```python
from build123d import *

# Parameters (mm, degrees)
SKETCH1_W           = 85
SKETCH1_H           = 70
SKETCH1_R           = 1.375
SKETCH1_R_2         = 4.125
SKETCH1_W_2         = 2.024682369
SKETCH1_H_2         = 6.385975888
SKETCH1_R_3         = 1.875
SKETCH1_R_4         = 2
SKETCH1_R_5         = 3
BOSS_EXTRUDE4_DEPTH = 10
SKETCH1_7_R         = 4.5
CUT_EXTRUDE2_DEPTH  = 6
SKETCH1_11_R        = 4.5
SKETCH1_11_R_2      = 3
CUT_EXTRUDE10_DEPTH = 8


with BuildPart() as part:
    # Sketch1 → Boss-Extrude4 (new body)
    with BuildSketch(Plane(origin=(0, 0, 0), x_dir=(1, 0, 0), z_dir=(0, 1, 0))):
        with Locations((-9.775924906, 0)):
            Rectangle(SKETCH1_W, SKETCH1_H)
        with Locations((-37.275924906, -25)):
            Circle(SKETCH1_R, mode=Mode.SUBTRACT)
        with Locations((12.724075094, -25)):
            Circle(SKETCH1_R, mode=Mode.SUBTRACT)
        with Locations((-25.024682369, 0)):
            Circle(SKETCH1_R_2, mode=Mode.SUBTRACT)
        with Locations((-18.012341185, 0)):
            Rectangle(SKETCH1_W_2, SKETCH1_H_2, mode=Mode.SUBTRACT)
        with Locations((-37.275924906, 25)):
            Circle(SKETCH1_R, mode=Mode.SUBTRACT)
        with Locations((12.724075094, 25)):
            Circle(SKETCH1_R, mode=Mode.SUBTRACT)
        with Locations((0, 17.5)):
            Circle(SKETCH1_R_3, mode=Mode.SUBTRACT)
        with Locations((0, -17.5)):
            Circle(SKETCH1_R_4, mode=Mode.SUBTRACT)
        with Locations((7, 0)):
            Circle(SKETCH1_R_5, mode=Mode.SUBTRACT)
    extrude(amount=BOSS_EXTRUDE4_DEPTH)

    # Sketch1_7 → Cut-Extrude2 (cut)
    with BuildSketch(Plane(origin=(0, 0, 0), x_dir=(1, 0, 0), z_dir=(0, 1, 0))):
        with BuildLine():
            Line((3.625, 17.5), (3.625, 13.729507457))
            ThreePointArc((3.625, 13.729507457), (14.2, 0), (3.625, -13.729507457))
            Line((3.625, -13.729507457), (3.625, -17.5))
            ThreePointArc((3.625, -17.5), (0, -21.125), (-3.625, -17.5))
            Line((-3.625, -17.5), (-3.625, -13.729507457))
            ThreePointArc((-3.625, -13.729507457), (-8.669470541, -11.246345208), (-12.354756169, -7))
            Line((-12.354756169, -7), (-17, -7))
            Line((-17, -7), (-17, 7))
            Line((-17, 7), (-12.354756169, 7))
            ThreePointArc((-12.354756169, 7), (-8.669470541, 11.246345208), (-3.625, 13.729507457))
            Line((-3.625, 13.729507457), (-3.625, 17.5))
            ThreePointArc((-3.625, 17.5), (0, 21.125), (3.625, 17.5))
        make_face()
        with Locations((7, 0)):
            Circle(SKETCH1_7_R, mode=Mode.SUBTRACT)
    extrude(amount=CUT_EXTRUDE2_DEPTH, mode=Mode.SUBTRACT)

    # Sketch1_11 → Cut-Extrude10 (cut)
    with BuildSketch(Plane(origin=(0, 0, 0), x_dir=(1, 0, 0), z_dir=(0, 1, 0))):
        with Locations((7, 0)):
            Circle(SKETCH1_11_R)
        with Locations((7, 0)):
            Circle(SKETCH1_11_R_2, mode=Mode.SUBTRACT)
    extrude(amount=CUT_EXTRUDE10_DEPTH, mode=Mode.SUBTRACT)


solid = part.part
```
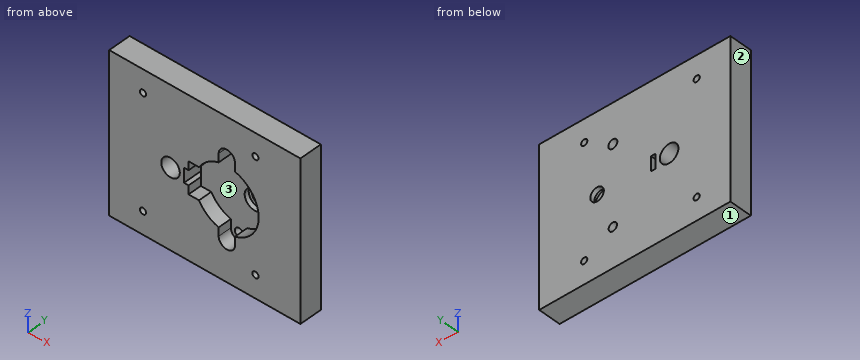
The model under review builds one solid part; all positions refer to its coordinate system, in mm. Face numbers are marked on the shaded views. Round coordinates to 2 decimals unless told otherwise and drop trailing zeros. Write each loop counter-clockwise with the first axis right and the second up, starting at its lowest first coordinate (ties: lowest second). Pieces come first, ordered by that corner, then holes. Notation, with made-up numbers: (39, 57) -> (53, 57) arc R5 cw to (53, 64) -> close; hole circle Ø11 at (-30, 26). An arc over 180 degrees is marked (long way). Use CSV: the item, a comma, the result in double quotes.
Q1. Consider section C-C (y = 4.25). State how many separate pieces and enclosed holes the cut face has, then the cut area to 3 significant figures.
Checks:
separate pieces,"1"
enclosed holes,"6"
area,"5,090 mm²"
Q2. Mouldability with a two-part tool opening along X and no side actions: class the marked faces 1, 2 and 3 as released by +X, released by -X, zero draft, split by the parting line, or undercut.
Checks:
face 1,"zero draft"
face 2,"released by -X"
face 3,"undercut"
Q3. Consider section A-A (x = 0). Give the boundary of the cut face in (y, z) (3 decimals), then the cut area to 4 significant figures.
Checks:
outline,"(0, -35) -> (10, -35) -> (10, -19.375) -> (6, -19.375) -> (6, -21.125) -> (0, -21.125) -> close; (0, 21.125) -> (6, 21.125) -> (6, 19.5) -> (10, 19.5) -> (10, 35) -> (0, 35) -> close; (6, -15.625) -> (10, -15.625) -> (10, 15.5) -> (6, 15.5) -> close"
area,"415.5 mm²"
Q4. Consider section B-B (z = 25). Give the boundary of the cut face in (x, y).
Checks:
outline,"(-52.28, 0) -> (-38.65, 0) -> (-38.65, 10) -> (-52.28, 10) -> close; (-35.9, 0) -> (11.35, 0) -> (11.35, 10) -> (-35.9, 10) -> close; (14.1, 0) -> (32.72, 0) -> (32.72, 10) -> (14.1, 10) -> close"
Q5. Consider section D-D (x = -14). Give the boundary of the cut face in (y, z), then the cut area to 3 significant figures.
Checks:
outline,"(0, -35) -> (10, -35) -> (10, 35) -> (0, 35) -> (0, 7) -> (6, 7) -> (6, -7) -> (0, -7) -> close"
area,"616 mm²"
Q6. For pin 1 Ø7 at (x, z) = (9, -1) entering from -Y, flat-tipped, find the tip position at first contact; note if it passes through.
Checks:
pin 1,"y = 6"
Q7. To check wall thickness, follow probe 1 along X at (y, z) = (7.5, 0); probe 2 along Z at (x, y) = (0, 8.2) (3 decimals); probe 3 along X at (y, z) = (3, 25). State the ranges of each line that lie inside material, in increasing order. Write a range as [from, to].
Checks:
probe 1,"[-52.28, -29.15], [-20.9, -19.02], [-17, 2.5], [11.5, 32.72]"
probe 2,"[-35, -19.375], [-15.625, 15.5], [19.5, 35]"
probe 3,"[-52.28, -38.65], [-35.9, 11.35], [14.1, 32.72]"
